Verification items for this drawing (mm, ordinates from the low corner). Round coordinates to 2 decimals unless told otherwise and drop trailing zeros. Write each loop counter-clockwise with the first axis right and the second up, starting at its lowest first coordinate (ties: lowest second). Pieces come first, ordered by that corner, then holes. Notation, with made-up numbers: (76, 82) -> (88, 82) arc R19 cw to (88, 86) -> close; hole circle Ø10 at (44, 88). An arc over 180 degrees is marked (long way). One line per question, with ' | ' between items.
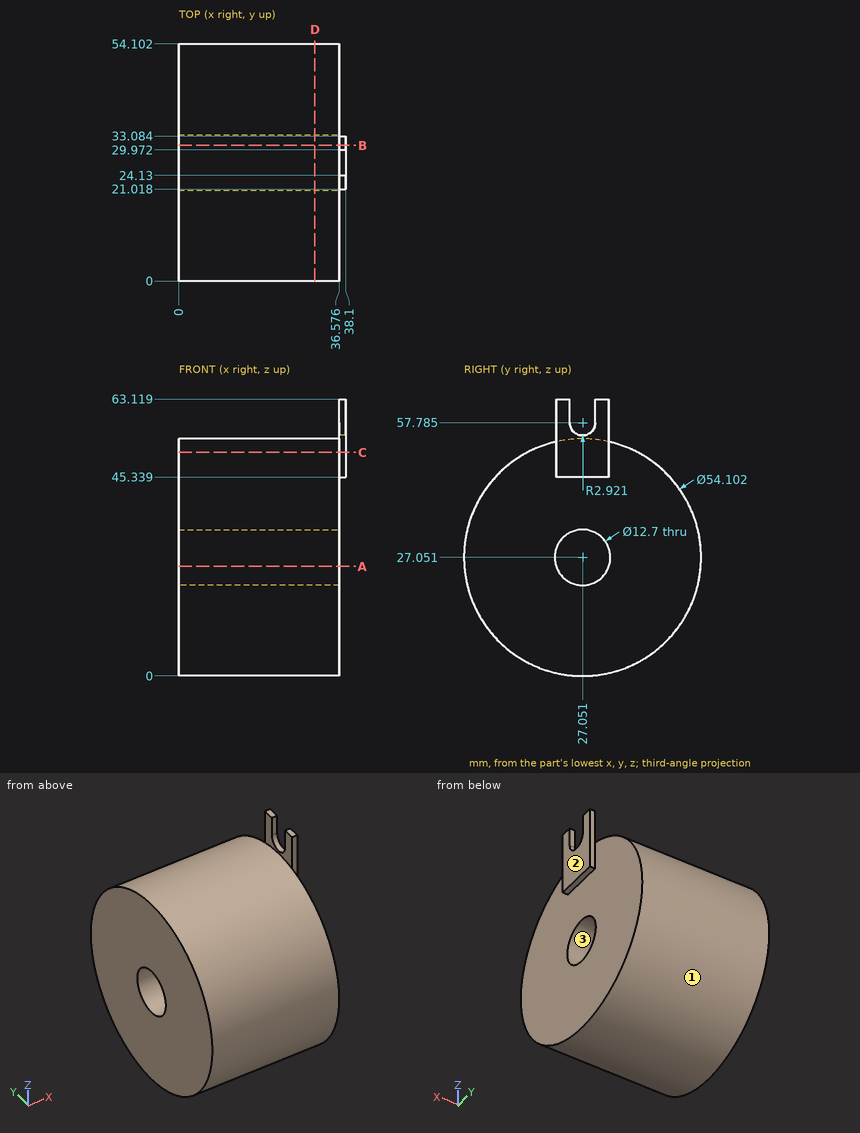
(1) Go/stop test with flat-tipped pins: pin 1 (1.2 mm diameter, centred on x = 37, y = 28, fed in from -Z) (1 decimal); pin 2 (10 mm diameter, centred on x = 4.5, z = 37.5, fed in from +Y); pin 3 (6 mm diameter, centred on x = 21.5, y = 45, fed in from +Z) (1 decimal). Record where each tip stops, or that it passes through.
Resolved:
pin 1: stops at z = 0 | pin 2: stops at y = 53.55 | pin 3: stops at z = 49.6
(2) Draft check along Z on the marked faces 1, 2 and 3. Enter one of: +Z half, -Z half, draft (parallel to the pull), parting line (faces both ways), or undercut.
Resolved:
face 1: parting line | face 2: draft | face 3: undercut
(3) Material ranges on line 1 (Z direction, x = 3, y = 27); line 2 (X direction, y = 20, z = 3) (1 decimal); line 3 (Z direction, x = 3.5, y = 31) (1 decimal), recorded low to high.
Resolved:
line 1: z = 0 to 20.7, 33.4 to 54.1 | line 2: x = 0 to 36.6 | line 3: z = 0.3 to 22.1, 32 to 53.8
(4) Sectioned sample at C-C on z = 51. Record the cut outline in (x, y) (1 decimal).
Resolved:
outline: (0, 14.5) -> (36.6, 14.5) -> (36.6, 21) -> (38.1, 21) -> (38.1, 33.1) -> (36.6, 33.1) -> (36.6, 39.6) -> (0, 39.6) -> close
(5) Sectioned sample at A-A on z = 25. Record the cut outline in (x, y) (1 decimal), then the cut area to 3 significant figures.
Resolved:
outline: (0, 0.1) -> (36.6, 0.1) -> (36.6, 21) -> (0, 21) -> close; (0, 33.1) -> (36.6, 33.1) -> (36.6, 54) -> (0, 54) -> close | area: 1,530 mm2
(6) Sectioned sample at D-D on x = 31. Record the cut outline in (y, z).
Resolved:
outline: circle Ø54.1 at (27.05, 27.05); hole circle Ø12.7 at (27.05, 27.05)
(7) Sectioned sample at B-B on y = 31. Record the cut outline in (x, z) (1 decimal).
Resolved:
outline: (0, 0.3) -> (36.6, 0.3) -> (36.6, 22.1) -> (0, 22.1) -> close; (0, 32) -> (36.6, 32) -> (36.6, 45.3) -> (38.1, 45.3) -> (38.1, 63.1) -> (36.6, 63.1) -> (36.6, 53.8) -> (0, 53.8) -> close
